```python
from build123d import *

# Parameters (mm, degrees)
SKETCH2_R           = 22.5
BOSS_EXTRUDE1_DEPTH = 3
BOSS_EXTRUDE2_DEPTH = 5
FILLET1_R           = 1
FILLET2_R           = 0.5
SKETCH5_R           = 3
CUT_EXTRUDE1_DEPTH  = 5


with BuildPart() as part:
    # Sketch2 → Boss-Extrude1 (new body)
    with BuildSketch(Plane(origin=(0, 0, 0), x_dir=(1, 0, 0), z_dir=(0, 1, 0))):
        with Locations(Location((0, 0, 0), (0, 0, 270))):
            Circle(SKETCH2_R)
    extrude(amount=BOSS_EXTRUDE1_DEPTH)

    # Sketch3 → Boss-Extrude2 (add)
    with BuildSketch(Plane(origin=(0, 3, 0), x_dir=(1, 0, 0), z_dir=(0, 1, 0))):
        with BuildLine():
            ThreePointArc((-4, 13.416407865), (-9.899494937, 9.899494937), (-13.416407865, 4))
            Line((-13.416407865, 4), (-8.062257748, 4))
            ThreePointArc((-8.062257748, 4), (-6.363961031, 6.363961031), (-4, 8.062257748))
            Line((-4, 8.062257748), (-4, 13.416407865))
        make_face()
        with BuildLine():
            ThreePointArc((13.416407865, 4), (9.899494937, 9.899494937), (4, 13.416407865))
            Line((4, 13.416407865), (4, 8.062257748))
            ThreePointArc((4, 8.062257748), (6.363961031, 6.363961031), (8.062257748, 4))
            Line((8.062257748, 4), (13.416407865, 4))
        make_face()
        with BuildLine():
            Line((4, -8.062257748), (4, -13.416407865))
            ThreePointArc((4, -13.416407865), (9.899494937, -9.899494937), (13.416407865, -4))
            Line((13.416407865, -4), (8.062257748, -4))
            ThreePointArc((8.062257748, -4), (6.363961031, -6.363961031), (4, -8.062257748))
        make_face()
        with BuildLine():
            Line((-8.062257748, -4), (-13.416407865, -4))
            ThreePointArc((-13.416407865, -4), (-9.899494937, -9.899494937), (-4, -13.416407865))
            Line((-4, -13.416407865), (-4, -8.062257748))
            ThreePointArc((-4, -8.062257748), (-6.363961031, -6.363961031), (-8.062257748, -4))
        make_face()
    extrude(amount=BOSS_EXTRUDE2_DEPTH)

    # Fillet1
    fillet1_edges = [part.edges().sort_by_distance(p)[0] for p in [
        (-6.363961031, 3, -6.363961031),
        (-4, 3, -10.739332807),
        (4, 5.5, -8.062257748),
        (10.739332807, 3, -4),
        (8.062257748, 5.5, -4),
        (4, 3, -10.739332807),
        (6.363961031, 3, -6.363961031),
        (8.062257748, 5.5, 4),
        (4, 3, 10.739332807),
        (4, 5.5, 8.062257748),
        (6.363961031, 3, 6.363961031),
        (10.739332807, 3, 4),
        (-4, 5.5, 8.062257748),
        (-8.062257748, 5.5, 4),
        (-6.363961031, 3, 6.363961031),
        (-4, 3, 10.739332807),
        (-10.739332807, 3, 4),
        (-8.062257748, 5.5, -4),
        (-4, 5.5, -8.062257748),
        (-10.739332807, 3, -4),
    ]]
    fillet(fillet1_edges, radius=FILLET1_R)

    # Fillet2
    fillet2_edges = [part.edges().sort_by_distance(p)[0] for p in [
        (9.899494937, 8, -9.899494937),
        (9.899494937, 8, 9.899494937),
        (-9.899494937, 8, 9.899494937),
        (-9.899494937, 8, -9.899494937),
    ]]
    fillet(fillet2_edges, radius=FILLET2_R)

    # Sketch5 → Cut-Extrude1 (cut)
    with BuildSketch(Plane(origin=(0, 3, 0), x_dir=(1, 0, 0), z_dir=(0, 1, 0))):
        with Locations(Location((0, 5, 0), (0, 0, 270))):
            Circle(SKETCH5_R)
    extrude(amount=-CUT_EXTRUDE1_DEPTH, mode=Mode.SUBTRACT)


solid = part.part
```
Can you work these out from the model? Positions are in its coordinate system, mm. A direction names the side the tool comes from. Coordinates: 2 decimals unless noted, no trailing zeros. Order: outer loops, then holes, each group sorted by start corner. A loop starts at its lowest first (then second) coordinate and runs counter-clockwise, first axis right, second up.
1. I'm going to push flat-ended pins straight in: pin 1 (4.5 mm diameter, centred on y = 6.5, z = 10.5, fed in from +X); pin 2 (4.5 mm diameter, centred on x = 11, y = 6.5, fed in from +Z); pin 3 (2 mm diameter, centred on y = 5.5, z = -10.5, fed in from -X); pin 4 (5 mm diameter, centred on x = 0, z = -5, fed in from -Y). Where does each tip first touch, or does it pass through?
2. If we section it at C-C (z = 0): Please give me the cut outline in (x, y).
3. If we section it at B-B (y = 1.75): Please give me the cut outline in (x, z), then the cut area to 3 significant figures.
4. Thinking about a two-plate mould opening in Z: for faces 1 (the face through (6.34, 5.97, -6.39)), 2 (the face through (-8.618, 1.479, 20.784)), 3 (the face through (4, 6, 11)), which applies, +Z half, -Z half, draft (parallel to the pull), parting line (faces both ways), or undercut?
5. If we section it at A-A (y = 6.25): Please give me the cut outline in (x, z), then the cut area to 3 significant figures.
6. If we section it at D-D (x = 16): Please give me the cut outline in (y, z), then the cut area to 3 significant figures.
7. I need wall thicknesses on line 1 (Y direction, x = 13, z = 1.5); line 2 (Z direction, x = -7.5, y = 5.75); line 3 (X direction, y = 3.5, z = -5). Which ranges of each line are inside material? Lowest first, please.
8. For faces 4 (the face through (-3.699, 3.285, -11.203)), 5 (the face through (10, 5.2, -9.8)), 6 (the face through (-6.39, 5.97, -6.34)), which set-ups out of +Z, -Z, +X, -X, +Y, -Y let a thin tool reach every point of the face, with its end or its side?
Entries:
1. pin 1: stops at x = 11.31
1. pin 2: stops at z = 10.93
1. pin 3: stops at x = -10.28
1. pin 4: passes through
2. outline: (-22.5, 0) - (22.5, 0) - (22.5, 3) - (-22.5, 3) - close
3. outline: circle Ø45 at (0, 0); hole circle Ø6 at (0, -5)
3. area: 1,560 mm2
4. face 1: undercut
4. face 2: parting line
4. face 3: draft
5. outline: (-13.42, -4) arc R14 ccw to (-4, -13.42) - (-4, -8.66) arc R1 ccw to (-4.5, -7.79) arc R9 cw to (-7.79, -4.5) arc R1 ccw to (-8.66, -4) - close; (-13.42, 4) - (-8.66, 4) arc R1 ccw to (-7.79, 4.5) arc R9 cw to (-4.5, 7.79) arc R1 ccw to (-4, 8.66) - (-4, 13.42) arc R14 ccw to start; (4, -13.42) arc R14 ccw to (13.42, -4) - (8.66, -4) arc R1 ccw to (7.79, -4.5) arc R9 cw to (4.5, -7.79) arc R1 ccw to (4, -8.66) - close; (4, 8.66) arc R1 ccw to (4.5, 7.79) arc R9 cw to (7.79, 4.5) arc R1 ccw to (8.66, 4) - (13.42, 4) arc R14 ccw to (4, 13.42) - close
5. area: 197 mm2
6. outline: (0, -15.82) - (3, -15.82) - (3, 15.82) - (0, 15.82) - close
6. area: 94.9 mm2
7. line 1: y = 0 to 3
7. line 2: z = -11.82 to -4.97, 4.97 to 11.82
7. line 3: x = -13.08 to -7.32, 7.32 to 13.08
8. face 4: +Z, -Z, +Y
8. face 5: -Z, +X, +Y
8. face 6: +Y
